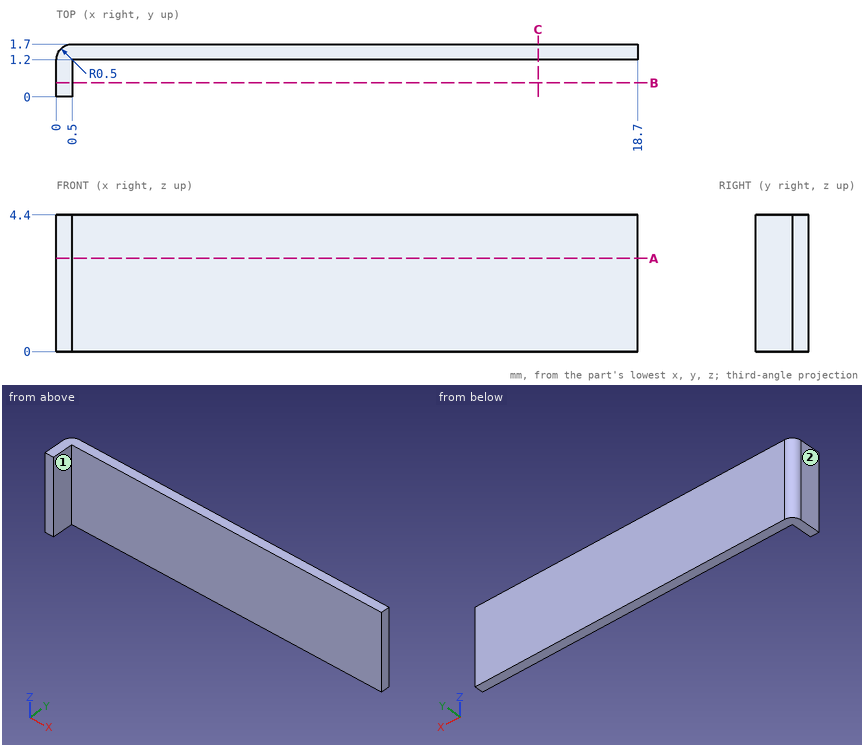
The drawing under review shows one solid part. Ordinate dimensions are in mm from its lowest x, y, z. A direction names the side the tool comes from. Round coordinates to 2 decimals unless told otherwise and drop trailing zeros. Loops run counter-clockwise (first coordinate to the right, second up) from the corner with the lowest first, then second, coordinate; pieces in that order, holes last. Notation, with made-up numbers: (-5, -18.5) - (21, -18.5) arc R22 cw to (21, -8.5) - close; hole circle Ø11 at (-29.75, -19.75). An arc over 180 degrees is marked (long way). One line per item, written item: value. Start each with the question number.
1) Consider section C-C on x = 15.5. Give the boundary of the cut face in (y, z), then the cut area to 3 significant figures.
2) For the marked faces 1 and 2, list the 3-axis set-ups (+Z, -Z, +X, -X, +Y, -Y) from which the entire face can be reached by the end or side of a thin tool; tool diameter is ignored.
3) Insertion check: pin 1 Ø1.3 at (x, z) = (5.5, 1.5) entering from -Y. The pin has a flat end and moves straight along its axis. Give the tip position at first contact, or say it passes through.
4) To check wall thickness, follow L1, parallel to X at y = 1.05, z = 3.65; L2, parallel to Y at x = 12, z = 0.4; L3, parallel to X at y = 1.25, z = 4.25. State the ranges of each line that lie inside material, in increasing order. Write a range as from..to.
5) Consider section B-B on y = 0.45. Give the boundary of the cut face in (x, z).
6) Consider section A-A on z = 3. Give the boundary of the cut face in (x, y), then the cut area to 3 significant figures.
Reported:
1. outline: (1.2, 0) - (1.7, 0) - (1.7, 4.4) - (1.2, 4.4) - close
1. area: 2.20 mm^2
2. face 1: +Z, -Z, +X, -Y
2. face 2: +Z, -Z, -X, +Y, -Y
3. pin 1: stops at y = 1.2
4. L1: x = 0..0.5
4. L2: y = 1.2..1.7
4. L3: x = 0..18.7
5. outline: (0, 0) - (0.5, 0) - (0.5, 4.4) - (0, 4.4) - close
6. outline: (0, 0) - (0.5, 0) - (0.5, 1.2) - (18.7, 1.2) - (18.7, 1.7) - (0.5, 1.7) arc R0.5 ccw to (0, 1.2) - close
6. area: 9.90 mm^2
